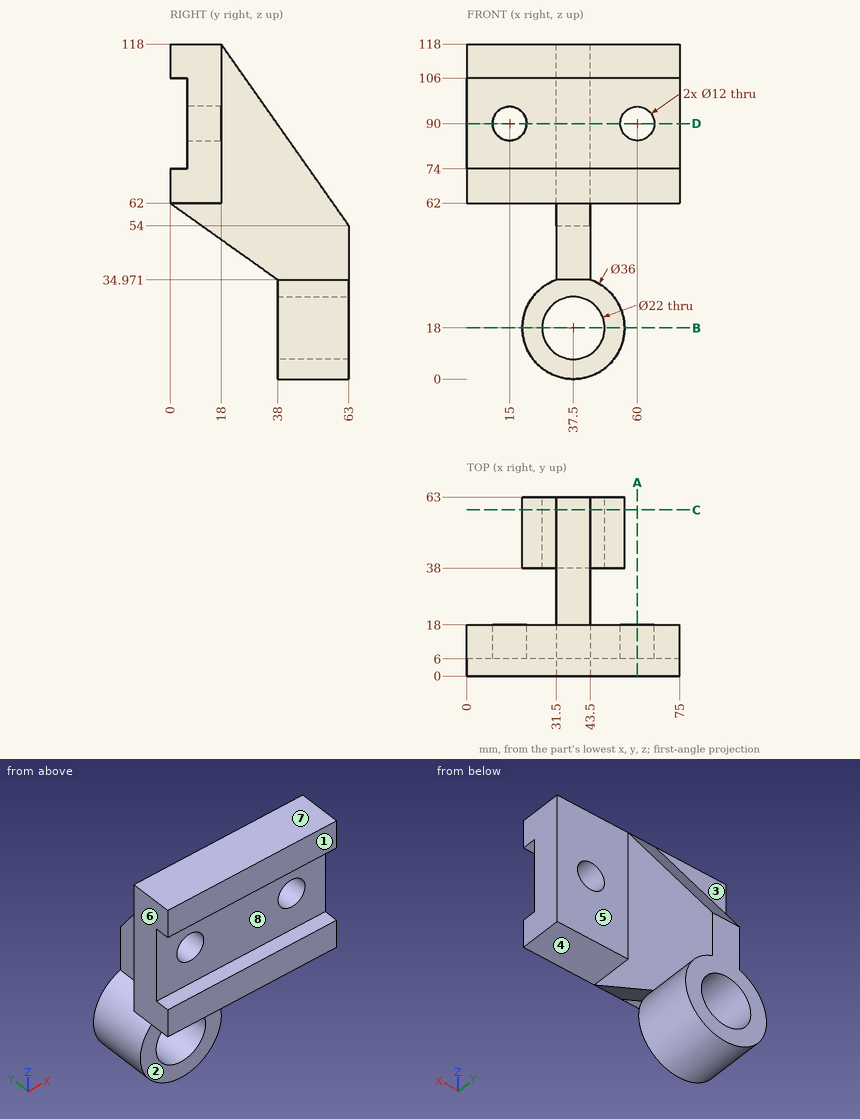
Print and shaded views of the part. All mm, measured from the part's lowest x, y and z. A direction names the side the tool comes from. Give positions to 0.01 mm unless a question says otherwise; leave off trailing zeros. Order: outer loops, then holes, each group sorted by start corner. A loop starts at its lowest first (then second) coordinate and runs counter-clockwise, first axis right, second up. Notation, with made-up numbers: (28.5, 26) - (78.5, 26) arc R32 cw to (78.5, 52) - close; hole circle Ø9 at (85.5, -15.5). An arc over 180 degrees is marked (long way). One line per item, written item: value.
Item 1: Tool access for the marked faces 1, 2, 3, 4 and 5: list every direction of +Z, -Z, +X, -X, +Y, -Y with a clear straight run to the whole face (end or side of a thin tool).
Response values:
face 1: +Z, -Z, +X, -X, -Y
face 2: -Z, +X, -X, -Y
face 3: +Z, -Z, -X, +Y
face 4: -Z, +X, +Y, -Y
face 5: +Z, -Z, +X, +Y
Item 2: Slice it at C-C (y = 58.5). List the corners of the cut face in (x, z).
Response values:
outline: (31.5, 34.97) arc R18 ccw (long way) to (43.5, 34.97) - (43.5, 60.4) - (31.5, 60.4) - close; hole circle Ø22 at (37.5, 18)
Item 3: Slice it at D-D (z = 90). List the corners of the cut face in (x, y), then the cut area to 3 significant figures.
Response values:
outline: (0, 6) - (9, 6) - (9, 18) - (0, 18) - close; (21, 6) - (54, 6) - (54, 18) - (43.5, 18) - (43.5, 37.69) - (31.5, 37.69) - (31.5, 18) - (21, 18) - close; (66, 6) - (75, 6) - (75, 18) - (66, 18) - close
area: 848 mm2
Item 4: Wall check: line 1 (X direction, y = 11.25, z = 90); line 2 (X direction, y = 7, z = 94); line 3 (X direction, y = 54, z = 18). Give the ranges that are in metal, low to high.
Response values:
line 1: 0 to 9, 21 to 54, 66 to 75
line 2: 0 to 10.53, 19.47 to 55.53, 64.47 to 75
line 3: 19.5 to 26.5, 48.5 to 55.5
Item 5: Pin check, flat tips, straight feed: pin 1 Ø15.5 at (x, z) = (15, 90) entering from +Y; pin 2 Ø20 at (x, y) = (9, 5) entering from -Z; pin 3 Ø3 at (y, z) = (33, 38) entering from -X. Stop position of each tip, or through.
Response values:
pin 1: y = 18
pin 2: z = 62
pin 3: x = 31.5
Item 6: Two-plate mould, pull along Z, no slides. Class the marked faces 6, 7 and 8: released by +Z, released by -Z, zero draft, split by the parting line, or undercut.
Response values:
face 6: zero draft
face 7: released by +Z
face 8: undercut
Item 7: Slice it at B-B (z = 18). List the corners of the cut face in (x, y), then the cut area to 3 significant figures.
Response values:
outline: (19.5, 38) - (26.5, 38) - (26.5, 63) - (19.5, 63) - close; (48.5, 38) - (55.5, 38) - (55.5, 63) - (48.5, 63) - close
area: 350 mm2
Item 8: Slice it at A-A (x = 60). List the corners of the cut face in (y, z), then the cut area to 3 significant figures.
Response values:
outline: (0, 62) - (18, 62) - (18, 84) - (6, 84) - (6, 74) - (0, 74) - close; (0, 106) - (6, 106) - (6, 96) - (18, 96) - (18, 118) - (0, 118) - close
area: 672 mm2
